Job drawing, mm, ordinate dimensions from the low corner. One solid piece. A direction names the side the tool comes from. Round coordinates to 2 decimals unless told otherwise and drop trailing zeros. Order: outer loops, then holes, each group sorted by start corner. A loop starts at its lowest first (then second) coordinate and runs counter-clockwise, first axis right, second up. Notation, with made-up numbers: (2.25, 48.5) - (25.25, 48.5) arc R22 cw to (25.25, 62.5) - close; hole circle Ø3 at (57.25, 22.25). An arc over 180 degrees is marked (long way). Use one line per item in the form item = value. Start each with the question number.
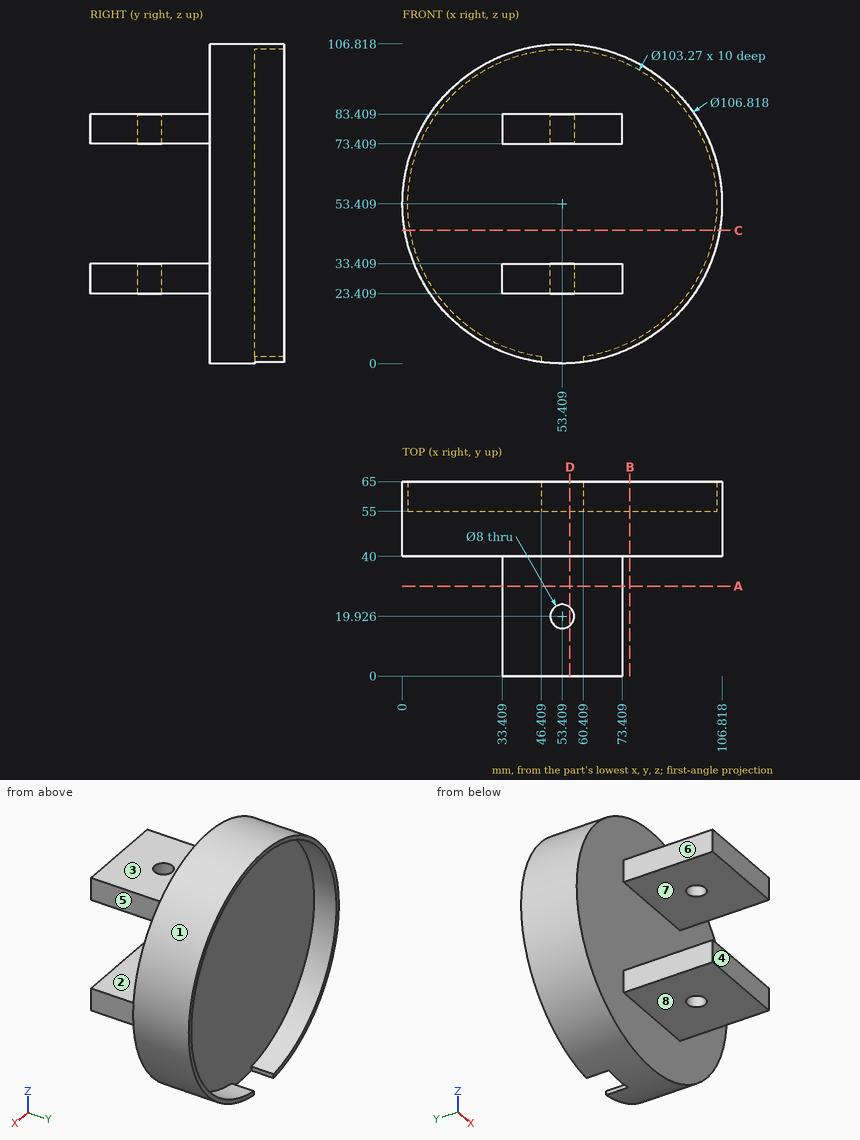
(1) Mould opens along Z. For the marked faces 1, 2, 3 and 4 say: pulls with the +Z half, pulls with the -Z half, needs draft (parallel to the pull), parting line crosses it, or undercut.
(2) Slice it at A-A (y = 30). Give the cut face in (x, z), and give its area (3 significant figures).
(3) Slice it at C-C (z = 44.5). Give the cut face in (x, y), and give its area (3 significant figures).
(4) Slice it at B-B (x = 76). Give the cut face in (y, z) (1 decimal), and give its area (3 significant figures).
(5) Flat gauge pins, fed straight in: P1, Ø8, axis at y = 20, z = 27.5, coming from the +X side; P2, Ø7, axis at x = 53.41, y = 19.93, coming from the -Z side; P3, Ø1.5, axis at x = 69.5, z = 65, coming from the -Y side; P4, Ø6, axis at x = 58.5, y = 34, coming from the +Z side. Where does each tip first touch, or does it go through?
(6) Slice it at D-D (x = 56). Give the cut face in (y, z) (1 decimal).
(7) Wall check: line 1 (Z direction, x = 56, y = 16); line 2 (Y direction, x = 30, z = 72.5); line 3 (Y direction, x = 58, z = 74.5). Give the ranges that are in metal, low to high. Write a range as [from, to].
(8) Which spindle directions (+Z, -Z, +X, -X, +Y, -Y) get a long thin tool onto all of the face, cutting with end or side? Do the marked faces 5, 6, 7 and 8. Say none if no direction does.
Results list:
q1.face_1 = parting line crosses it
q1.face_2 = undercut
q1.face_3 = pulls with the +Z half
q1.face_4 = needs draft
q2.outline = (33.41, 23.41) - (73.41, 23.41) - (73.41, 33.41) - (33.41, 33.41) - close; (33.41, 73.41) - (73.41, 73.41) - (73.41, 83.41) - (33.41, 83.41) - close
q2.area = 800 mm²
q3.outline = (0.75, 40) - (106.07, 40) - (106.07, 65) - (104.27, 65) - (104.27, 55) - (2.55, 55) - (2.55, 65) - (0.75, 65) - close
q3.area = 1,620 mm²
q4.outline = (40, 5) - (65, 5) - (65, 7) - (55, 7) - (55, 99.8) - (65, 99.8) - (65, 101.8) - (40, 101.8) - close
q4.area = 1,490 mm²
q5.P1 = 73.41
q5.P2 = through
q5.P3 = 40
q5.P4 = 83.41
q6.outline = (0, 23.4) - (16.9, 23.4) - (16.9, 33.4) - (0, 33.4) - close; (0, 73.4) - (16.9, 73.4) - (16.9, 83.4) - (0, 83.4) - close; (23, 23.4) - (40, 23.4) - (40, 0.1) - (55, 0.1) - (55, 105) - (65, 105) - (65, 106.8) - (40, 106.8) - (40, 83.4) - (23, 83.4) - (23, 73.4) - (40, 73.4) - (40, 33.4) - (23, 33.4) - close
q7.line_1 = [23.41, 33.41], [73.41, 83.41]
q7.line_2 = [40, 55]
q7.line_3 = [0, 55]
q8.face_5 = +Z, -Z, +X, -Y
q8.face_6 = +Z, -Z, -X, -Y
q8.face_7 = +X, -X, -Y
q8.face_8 = -Z, +X, -X, -Y
